Model file for the job. Use its own axes, mm. Give positions to 0.01 mm unless a question says otherwise; leave off trailing zeros. Order: outer loops, then holes, each group sorted by start corner. A loop starts at its lowest first (then second) coordinate and runs counter-clockwise, first axis right, second up. Notation, with made-up numbers: (14, -34.75) -> (72, -34.75) arc R11 cw to (72, -15.75) -> close; hole circle Ø1 at (63, 85). An arc over 180 degrees is marked (long way). Answer in a Markdown table with one row per item. Add a question column.
Autodesk Inventor part; units mm, degrees
ref_plane "YZ Plane" through (0, 0, 0) normal (1, 0, 0) x (0, 1, 0)
ref_plane "XZ Plane" through (0, 0, 0) normal (0, 1, 0) x (-1, 0, 0)
ref_plane "XY Plane" through (0, 0, 0) normal (0, 0, 1) x (1, 0, 0)
sketch "Sketch1" plane through (0, 0, 0) normal (0, 1, 0) x (-1, 0, 0)
  line L0 (24, 32) -> (-24, 32) construction
  line L1 (-24, 32) -> (-24, -32) construction
  line L2 (-24, -32) -> (24, -32) construction
  line L3 (24, -32) -> (24, 32) construction
  line L4 (24, 32) -> (-24, -32) construction
  line L5 (-24, 32) -> (24, -32) construction
  line L6 (26, 36) -> (-26, 36)
  line L7 (-28, 34) -> (-28, -34)
  line L8 (-26, -36) -> (26, -36)
  line L9 (28, -34) -> (28, 34)
  arc A0 (26, -36) -> (28, -34) centre (26, -34) ccw
  arc A1 (28, 34) -> (26, 36) centre (26, 34) ccw
  arc A2 (-26, 36) -> (-28, 34) centre (-26, 34) ccw
  arc A3 (-28, -34) -> (-26, -36) centre (-26, -34) ccw
  circle A4 centre (24, -32) radius 2.1
  circle A5 centre (-24, -32) radius 2.1
  circle A6 centre (-24, 32) radius 2.1
  circle A7 centre (24, 32) radius 2.1
  circle A8 centre (0, 0) radius 2.1
  dimension "d0" = 48
  dimension "d1" = 64
  dimension "d2" = 4
  dimension "d3" = 2
  dimension "d4" = 4.2
  dimension "d5" = 4.2
  dimension "d6" = 4.2
  dimension "d7" = 4.2
  dimension "d8" = 4.2
extrude "Extrusion1" add sketch "Sketch1" along normal blind 3
properties part number "StageConnectionPlate" material "Aluminum 6061"
Item 1: Saw through at B-B on x = 24. List the corners of the cut face in (y, z).
Item 2: Two-plate mould, pull along X, no slides. Class faces 1 (the cylindrical face through (23.031, 1.479, -30.137)), 2 (the flat face through (0, 1, 36)), 3 (the cylindrical face through (-27.43, 1.48, -35.4)): pulls with the +X half, pulls with the -X half, needs draft (parallel to the pull), parting line crosses it, or undercut.
Item 3: Pin check, flat tip, straight feed: pin 1 Ø1.5 at (x, z) = (-3, -10) entering from -Y. Stop position of the tip, or through.
Item 4: Wall check: line 1 (Z direction, x = 24, y = 2.1); line 2 (Z direction, x = 0, y = 0.9); line 3 (X direction, y = 2.5, z = 32.5). Give the ranges that are in metal, low to high.
Item 5: Saw through at A-A on z = -32. List the corners of the cut face in (x, y).
Item 6: Saw through at C-C on z = 0. List the corners of the cut face in (x, y), plus the area to 3 significant figures.
Item 7: Saw through at D-D on y = 0.75. List the corners of the cut face in (x, z), plus the area to 3 significant figures.
Evaluation:
| question | item | result |
|---|---|---|
| 1 | outline | (0, -36) -> (3, -36) -> (3, -34.1) -> (0, -34.1) -> close; (0, -29.9) -> (3, -29.9) -> (3, 29.9) -> (0, 29.9) -> close; (0, 34.1) -> (3, 34.1) -> (3, 36) -> (0, 36) -> close |
| 2 | face 1 | undercut |
| 2 | face 2 | needs draft |
| 2 | face 3 | pulls with the -X half |
| 3 | pin 1 | stops at y = 0 |
| 4 | line 1 | z = -36 to -34.1, -29.9 to 29.9, 34.1 to 36 |
| 4 | line 2 | z = -36 to -2.1, 2.1 to 36 |
| 4 | line 3 | x = -28 to -26.04, -21.96 to 21.96, 26.04 to 28 |
| 5 | outline | (-28, 0) -> (-26.1, 0) -> (-26.1, 3) -> (-28, 3) -> close; (-21.9, 0) -> (21.9, 0) -> (21.9, 3) -> (-21.9, 3) -> close; (26.1, 0) -> (28, 0) -> (28, 3) -> (26.1, 3) -> close |
| 6 | outline | (-28, 0) -> (-2.1, 0) -> (-2.1, 3) -> (-28, 3) -> close; (2.1, 0) -> (28, 0) -> (28, 3) -> (2.1, 3) -> close |
| 6 | area | 155 mm2 |
| 7 | outline | (-28, -34) arc R2 ccw to (-26, -36) -> (26, -36) arc R2 ccw to (28, -34) -> (28, 34) arc R2 ccw to (26, 36) -> (-26, 36) arc R2 ccw to (-28, 34) -> close; hole circle Ø4.2 at (-24, -32); hole circle Ø4.2 at (-24, 32); hole circle Ø4.2 at (0, 0); hole circle Ø4.2 at (24, -32); hole circle Ø4.2 at (24, 32) |
| 7 | area | 3,960 mm2 |
